Geometry check sheet. Reference: the model listing, model coordinates, mm. Face numbers are marked on the shaded views. A direction names the side the tool comes from. Give positions to 0.01 mm unless a question says otherwise; leave off trailing zeros. Order: outer loops, then holes, each group sorted by start corner. A loop starts at its lowest first (then second) coordinate and runs counter-clockwise, first axis right, second up.
```python
from build123d import *

# Parameters (mm, degrees)
PAD007_DEPTH       = 2
PAD010_DEPTH       = 3.5
POCKET003005_DEPTH = 2.25
SKETCH016_R        = 4.702209
PAD011_DEPTH       = 1.2
SKETCH017_R        = 3.711245
POCKET003006_DEPTH = 5
PAD014_DEPTH       = 3.5
SKETCH031_R        = 1.7
POCKET003015_DEPTH = 5
PAD019_DEPTH       = 4
POCKET003038_DEPTH = 3


with BuildPart() as part:
    # Sketch010 → Pad007 (new body, symmetric)
    with BuildSketch(Plane.XZ):
        with BuildLine():
            Line((0, 28.012352), (20.118014, 28.012352))
            ThreePointArc((27.996705, 20.985645), (25.39647, 26.000475), (20.118014, 28.012352))
            Line((27.996705, 20.985645), (30.977077, -4.999855))
            Line((33.977077, -4.999855), (30.977077, -4.999855))
            Line((31.375086, 21.001563), (33.977077, -4.999855))
            ThreePointArc((31.375086, 21.001563), (27.724484, 28.375327), (20.118014, 31.512352))
            Line((0, 31.512352), (20.118014, 31.512352))
            Line((0, 28.012352), (0, 31.512352))
        make_face()
    extrude(amount=PAD007_DEPTH, both=True)

    # Sketch011 → Pad010 (new body)
    with BuildSketch(Plane(origin=(0, 0, 31.512352), x_dir=(-1, 0, 0), z_dir=(0, 0, 1))):
        with BuildLine():
            Line((-18.002971, 2.001985), (0, 2.001985))
            ThreePointArc((0, -10), (6.000993, -3.999007), (0, 2.001985))
            Line((-19, -4), (0, -10))
            ThreePointArc((-18.002971, 2.001985), (-20.489406, -0.668781), (-19, -4))
        make_face()
    extrude(amount=-PAD010_DEPTH)

    # Sketch015 → Pocket003005 (cut)
    with BuildSketch(Plane(origin=(0, 0, 31.512352), x_dir=(-1, 0, 0), z_dir=(0, 0, 1))):
        with BuildLine():
            Line((-17.557616, 0.476904), (0, 0.476904))
            ThreePointArc((0.265399, -8.449899), (4.421634, -3.858985), (0, 0.476904))
            Line((0.265399, -8.449899), (-18.344393, -2.383287))
            ThreePointArc((-17.557616, 0.476904), (-18.678345, -0.753115), (-18.344393, -2.383287))
        make_face()
    extrude(amount=-POCKET003005_DEPTH, mode=Mode.SUBTRACT)

    # Sketch016 → Pad011 (new body)
    with BuildSketch(Plane(origin=(0, 0, 28.012352), x_dir=(1, 0, 0), z_dir=(0, 0, -1))):
        with Locations((-0.089106, -3.841625)):
            Circle(SKETCH016_R)
    extrude(amount=PAD011_DEPTH)

    # Sketch017 → Pocket003006 (cut)
    with BuildSketch(Plane(origin=(0, 0, 26.812352), x_dir=(1, 0, 0), z_dir=(0, 0, -1))):
        with Locations((-0.080471, -3.899184)):
            Circle(SKETCH017_R)
    extrude(amount=-POCKET003006_DEPTH, mode=Mode.SUBTRACT)

    # Sketch022 → Pad014 (new body)
    with BuildSketch(Plane(origin=(0, 0, 31.512352), x_dir=(-1, 0, 0), z_dir=(0, 0, 1))):
        with BuildLine():
            Line((-20.438215, -2), (-13.234047, -4.102969))
            Line((-13.234047, -4.102969), (-13.028216, -6.021869))
            Line((-13.028216, -6.021869), (-13.028216, -8.298126))
            ThreePointArc((-22.034031, -8.18918), (-17.561616, -10.764285), (-13.028216, -8.298126))
            Line((-22.034031, -8.18918), (-22.034031, -2))
            Line((-20.438215, -2), (-22.034031, -2))
        make_face()
    extrude(amount=-PAD014_DEPTH)

    # Sketch031 → Pocket003015 (cut)
    with BuildSketch(Plane(origin=(0, 0, 31.512352), x_dir=(-1, 0, 0), z_dir=(0, 0, 1))):
        with Locations((-17.509254, -6.500788)):
            Circle(SKETCH031_R)
    extrude(amount=-POCKET003015_DEPTH, mode=Mode.SUBTRACT)

    # Sketch032 → Pad019 (new body)
    with BuildSketch(Plane.XZ.offset(2)):
        with BuildLine():
            Line((27, 28.536497), (32.513573, -5))
            Line((32.513573, -5), (37.000002, -5))
            Line((37.000002, -5), (37.000002, -4.583553))
            ThreePointArc((33.505627, -1), (35.019116, -3.019659), (37.000002, -4.583553))
            Line((33, 5), (33.505627, -1))
            Line((35, 3.304739), (33, 5))
            Line((32.728943, 7), (35, 3.304739))
            Line((32, 13), (32.728943, 7))
            Line((34.496559, 10.608005), (32, 13))
            Line((32, 15), (34.496559, 10.608005))
            Line((31, 20), (32, 15))
            Line((33.606815, 17.606869), (31, 20))
            Line((31, 22), (33.606815, 17.606869))
            Line((27, 28.536497), (31, 22))
        make_face()
    extrude(amount=-PAD019_DEPTH)

    # Sketch074 → Pocket003038 (cut)
    with BuildSketch(Plane(origin=(0, 0, 31.512352), x_dir=(-1, 0, 0), z_dir=(0, 0, 1))):
        Polygon((-16.869587, -9.826502), (-14.299442, -7.600665), (-14.942, -4.261935), (-18.154705, -3.149042), (-20.72485, -5.374879), (-20.082292, -8.713609), align=None)
    extrude(amount=-POCKET003038_DEPTH, mode=Mode.SUBTRACT)


solid = part.part
```
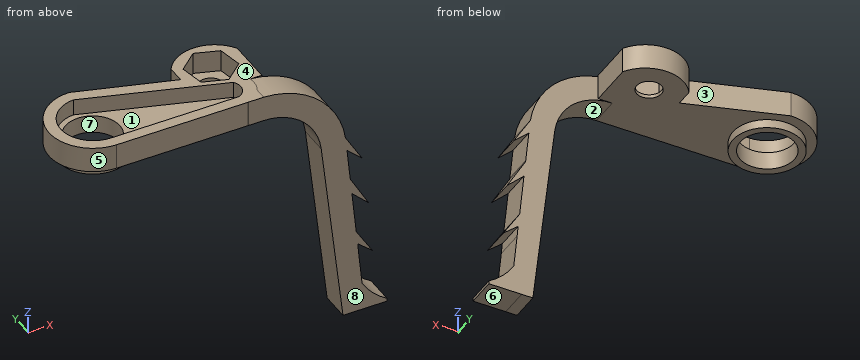
Q1. Thickness scan on L1, parallel to Z at x = 9.5, y = 0.5; L2, parallel to Z at x = 15, y = 4.5; L3, parallel to Y at x = 32, z = 5. Record the ranges inside material, lowest first.
Q2. Release check for a two-part mould opening along Y. For the marked faces 6, 7 and 8 record: pulls with the +Y half, pulls with the -Y half, needs draft (parallel to the pull), parting line crosses it, or undercut.
Q3. Access from +Z, -Z, +X, -X, +Y, -Y to the whole of each face (thin tool, end or side, straight path). Record for the marked faces 1, 2, 3, 4 and 5.
Q4. Cross-section at C-C, the plane z = 13.5. Record the boundary of the cut face in (x, y).
Q5. Cross-section at B-B, the plane z = 8. Record the boundary of the cut face in (x, y).
Q6. Cross-section at A-A, the plane x = 12. Record the boundary of the cut face in (y, z).
Q7. Gauge pin test, flat ends, axial feed: P1, Ø1.5, axis at x = 15, y = 1.5, coming from the -Z side; P2, Ø13.5, axis at x = 29, z = 5.5, coming from the +Y side; P3, Ø1.8, axis at y = 5, z = 29, coming from the +X side. Record the tip position at first contact, or that the pin passes through.
Answers follow:
1. L1: z = 28.01 to 29.26
1. L2: z = 28.01 to 28.51
1. L3: y = -2 to 2
2. face 6: needs draft
2. face 7: undercut
2. face 8: pulls with the -Y half
3. face 1: +Z
3. face 2: -Z, +Y, -Y
3. face 3: +Z, -Z, +Y
3. face 4: +Z, +X, -X, +Y, -Y
3. face 5: +Z, -Z, -X
4. outline: (28.86, -2) - (32.85, -2) - (32.85, 2) - (28.86, 2) - close
5. outline: (29.49, -2) - (32.68, -2) - (32.68, 2) - (29.49, 2) - close
6. outline: (-2, 28.01) - (6.21, 28.01) - (6.21, 31.51) - (4.45, 31.51) - (4.45, 29.26) - (-0.48, 29.26) - (-0.48, 31.51) - (-2, 31.51) - close
7. P1: stops at z = 28.01
7. P2: stops at y = 2
7. P3: stops at x = 22.03
